```python
from build123d import *

# Parameters (mm, degrees)
F0_R     = 28
F0_R_2   = 1.75
F1_DEPTH = 5
F2_R     = 13
F3_DEPTH = 3.5
F4_R     = 9
F5_DEPTH = 1.501


# Not quite as in the source:
# - a feature names something its author has since deleted; it is built from what else it names


with BuildPart() as f1:
    # F0 (on Top) → F1 (new body)
    with BuildSketch(Plane.XY):
        Circle(F0_R)
        with Locations((-20.75, -11.9800180857)):
            Circle(F0_R_2, mode=Mode.SUBTRACT)
        with Locations((20.75, -11.9800180857)):
            Circle(F0_R_2, mode=Mode.SUBTRACT)
        with Locations((0, 23.9600361714)):
            Circle(F0_R_2, mode=Mode.SUBTRACT)
    extrude(amount=F1_DEPTH)

    # F2 (on face) → F3 (cut)
    with BuildSketch(Plane.XY.offset(5)):
        Circle(F2_R)
    extrude(amount=-F3_DEPTH, mode=Mode.SUBTRACT)

    # F4 (on face) → F5 (cut, through all)
    with BuildSketch(Plane.XY.offset(1.5)):
        Circle(F4_R)
    extrude(amount=-F5_DEPTH, mode=Mode.SUBTRACT)


solid = f1.part
```
Build history of the part. All positions in model axes, mm. A direction names the side the tool comes from. Give positions to 0.01 mm unless a question says otherwise; leave off trailing zeros. Loops run counter-clockwise (first coordinate to the right, second up) from the corner with the lowest first, then second, coordinate; pieces in that order, holes last.
1) 3-axis set-ups, long thin cutter, end or side, ignore diameter. For faces 4 (the face through (-22.5, -11.9, 2.5)), 5 (the face through (-10.316, -7.91, 3.274)): which of +Z, -Z, +X, -X, +Y, -Y reach the whole face in a straight line?
Values follow:
face 4: +Z, -Z
face 5: +Z
2) Band-saw the part on A-A on y = 0. List the corners of the cut face in (x, z).
Values follow:
outline: (-28, 0) - (-9, 0) - (-9, 1.5) - (-13, 1.5) - (-13, 5) - (-28, 5) - close; (9, 0) - (28, 0) - (28, 5) - (13, 5) - (13, 1.5) - (9, 1.5) - close
3) Probe line 1 along Y through (x, z) = (0, 2.95); line 2 along Y through (x, z) = (0, 0.4); line 3 along Y through (x, z) = (-20.75, 3.8). List the from-to ranges inside material, lowest first.
Values follow:
line 1: y = -28 to -13, 13 to 22.21, 25.71 to 28
line 2: y = -28 to -9, 9 to 22.21, 25.71 to 28
line 3: y = -18.8 to -13.73, -10.23 to 18.8
4) Band-saw the part on C-C on x = 20.75. List the corners of the cut face in (y, z).
Values follow:
outline: (-18.8, 0) - (-13.73, 0) - (-13.73, 5) - (-18.8, 5) - close; (-10.23, 0) - (18.8, 0) - (18.8, 5) - (-10.23, 5) - close
5) Band-saw the part on D-D on z = 0.85. List the corners of the cut face in (x, y).
Values follow:
outline: circle Ø56 at (0, 0); hole circle Ø3.5 at (-20.75, -11.98); hole circle Ø18 at (0, 0); hole circle Ø3.5 at (0, 23.96); hole circle Ø3.5 at (20.75, -11.98)
6) Two-plate mould, pull along Y, no slides. Class faces 1 (the face through (3, 9, 1.5)), 2 (the face through (-7, 7, 0)), 3 (the face through (25.865, -10.724, 2.465)): released by +Y, released by -Y, zero draft, split by the parting line, or undercut.
Values follow:
face 1: undercut
face 2: zero draft
face 3: split by the parting line
7) Band-saw the part on B-B on x = 0. List the corners of the cut face in (y, z), then the cut area to 4 significant figures.
Values follow:
outline: (-28, 0) - (-9, 0) - (-9, 1.5) - (-13, 1.5) - (-13, 5) - (-28, 5) - close; (9, 0) - (22.21, 0) - (22.21, 5) - (13, 5) - (13, 1.5) - (9, 1.5) - close; (25.71, 0) - (28, 0) - (28, 5) - (25.71, 5) - close
area: 144.5 mm2
8) Drop flat-ended pins along their axis: P1, Ø11, axis at x = 0, y = 0, coming from the -Z side; P2, Ø1, axis at x = 20.5, z = 2, coming from the +Y side; P3, Ø21, axis at x = 1, y = 2, coming from the +Z side; P4, Ø1, axis at x = 5.5, z = 4, coming from the -Y side. Give the stop position or say it passes through.
Values follow:
P1: passes through
P2: stops at y = 19.6
P3: stops at z = 1.5
P4: stops at y = -27.55
